```python
from build123d import *

# Parameters (mm, degrees)
SKETCH1_W           = 225
SKETCH1_H           = 90
BOSS_EXTRUDE1_DEPTH = 43.8
BOSS_EXTRUDE2_DEPTH = 10


with BuildPart() as part:
    # Sketch1 → Boss-Extrude1 (new body)
    with BuildSketch(Plane.XY):
        Rectangle(SKETCH1_W, SKETCH1_H)
    extrude(amount=BOSS_EXTRUDE1_DEPTH)

    # Sketch2 → Boss-Extrude2 (add)
    with BuildSketch(Plane.XY):
        with BuildLine():
            Line((-112.5, 37), (-124.9, 37))
            ThreePointArc((-124.9, 37), (-125.607106781, 36.707106781), (-125.9, 36))
            Line((-125.9, 36), (-125.9, 23.25))
            ThreePointArc((-125.9, 23.25), (-125.607106781, 22.542893219), (-124.9, 22.25))
            Line((-124.9, 22.25), (-119.25, 22.25))
            ThreePointArc((-119.25, 22.25), (-117, 20), (-119.25, 17.75))
            Line((-119.25, 17.75), (-124.9, 17.75))
            ThreePointArc((-124.9, 17.75), (-125.607106781, 17.457106781), (-125.9, 16.75))
            Line((-125.9, 16.75), (-125.9, -16.75))
            ThreePointArc((-125.9, -16.75), (-125.607106781, -17.457106781), (-124.9, -17.75))
            Line((-124.9, -17.75), (-119.25, -17.75))
            ThreePointArc((-119.25, -17.75), (-117, -20), (-119.25, -22.25))
            Line((-119.25, -22.25), (-124.9, -22.25))
            ThreePointArc((-124.9, -22.25), (-125.607106781, -22.542893219), (-125.9, -23.25))
            Line((-125.9, -23.25), (-125.9, -36))
            ThreePointArc((-125.9, -36), (-125.607106781, -36.707106781), (-124.9, -37))
            Line((-124.9, -37), (-112.5, -37))
            Line((-112.5, -37), (-112.5, 37))
        make_face()
    boss_extrude2 = extrude(amount=BOSS_EXTRUDE2_DEPTH)

    # Mirror1: Boss-Extrude2 across plane
    add(boss_extrude2.mirror(Plane(origin=(0, 0, 0), x_dir=(0, 0, 1), z_dir=(1, 0, 0))))


solid = part.part
```
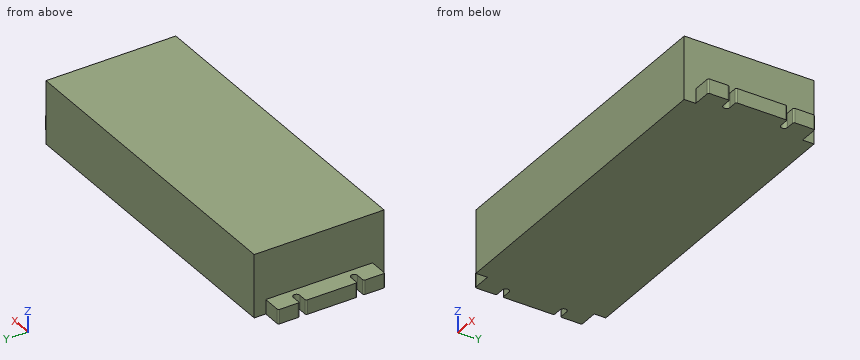
The listing builds one solid part. Answer for the finished solid, in the listing's coordinates (mm). Round coordinates to 2 decimals unless told otherwise and drop trailing zeros. Order: outer loops, then holes, each group sorted by start corner. A loop starts at its lowest first (then second) coordinate and runs counter-clockwise, first axis right, second up. Notation, with made-up numbers: (-39.75, 1) - (-14.75, 1) arc R23 ccw to (-14.75, 9) - close; hole circle Ø1 at (59.25, 2). An arc over 180 degrees is marked (long way). Put each result on its own line as item: value. Start each with the question number.
(1) Given P1, Ø6, axis at x = 121, z = 4, coming from the -Y side; P2, Ø4, axis at x = 120.5, y = 1, coming from the +Z side; P3, Ø8, axis at x = 116, z = 4, coming from the +Y side; P4, Ø2, axis at y = 31.5, z = 30.5, coming from the +X side, each flat-ended and moving along its own axis, determine where each tip first touches the part or whether it passes through.
(2) Find section B-B (z = 39.5). Give the vertices of the cut face in (x, y).
(3) A straight line is drawn through the part: probe 1 along X at (y, z) = (24.5, 24.5). Find the intervals that lie inside material, in ascending order. Write a range as from..to.
(4) Find section A-A (y = 27). Give the vertices of the cut face in (x, z), plus the area to 3 significant figures.
(5) Find section C-C (y = -20). Give the vertices of the cut face in (x, z), plus the area to 4 significant figures.
Reply:
1. P1: y = -37
1. P2: z = 10
1. P3: y = 45
1. P4: x = 112.5
2. outline: (-112.5, -45) - (112.5, -45) - (112.5, 45) - (-112.5, 45) - close
3. probe 1: -112.5..112.5
4. outline: (-125.9, 0) - (125.9, 0) - (125.9, 10) - (112.5, 10) - (112.5, 43.8) - (-112.5, 43.8) - (-112.5, 10) - (-125.9, 10) - close
4. area: 10,100 mm^2
5. outline: (-117, 0) - (117, 0) - (117, 10) - (112.5, 10) - (112.5, 43.8) - (-112.5, 43.8) - (-112.5, 10) - (-117, 10) - close
5. area: 9,945 mm^2
